Can you work these out from the model? Positions are in its coordinate system, mm. A direction names the side the tool comes from. Give positions to 0.01 mm unless a question says otherwise; leave off trailing zeros. Write each loop counter-clockwise with the first axis right and the second up, starting at its lowest first coordinate (ties: lowest second). Pieces come first, ordered by that corner, then holes. Notation, with made-up numbers: M -32,-39 L 17,-39 A24 ccw 17,-28 Z; hole C -34,79 d4. An arc over 180 degrees is marked long. Write each question's results on one line, items separated by ' | '.
from build123d import *

# Parameters (mm, degrees)
SKETCH1_W           = 101.6
SKETCH1_H           = 101.6
SKETCH1_W_2         = 4.7625
SKETCH1_H_2         = 8.89
SKETCH1_W_3         = 17.78
SKETCH1_H_3         = 50.8
SKETCH1_W_4         = 22.86
SKETCH1_H_4         = 6.35
BOSS_EXTRUDE1_DEPTH = 4.7625
FILLET1_R           = 5.08


with BuildPart() as part:
    # Sketch1 → Boss-Extrude1 (new body)
    with BuildSketch(Plane(origin=(0, 0, 0), x_dir=(1, 0, 0), z_dir=(0, 1, 0))):
        with Locations((-50.8, 50.8)):
            Rectangle(SKETCH1_W, SKETCH1_H)
        with Locations((-94.45625, 13.335)):
            Rectangle(SKETCH1_W_2, SKETCH1_H_2, mode=Mode.SUBTRACT)
        with Locations((-94.45625, 88.265)):
            Rectangle(SKETCH1_W_2, SKETCH1_H_2, mode=Mode.SUBTRACT)
        with Locations((-71.755, 50.8)):
            Rectangle(SKETCH1_W_3, SKETCH1_H_3, mode=Mode.SUBTRACT)
        with Locations((-36.195, 81.915)):
            Rectangle(SKETCH1_W_4, SKETCH1_H_4, mode=Mode.SUBTRACT)
        with Locations((-7.14375, 13.335)):
            Rectangle(SKETCH1_W_2, SKETCH1_H_2, mode=Mode.SUBTRACT)
        with Locations((-7.14375, 88.265)):
            Rectangle(SKETCH1_W_2, SKETCH1_H_2, mode=Mode.SUBTRACT)
        with Locations((-36.195, 34.925)):
            Rectangle(SKETCH1_W_4, SKETCH1_H_4, mode=Mode.SUBTRACT)
    extrude(amount=BOSS_EXTRUDE1_DEPTH)

    # Fillet1
    fillet1_edges = [part.edges().sort_by_distance(p)[0] for p in [
        (0, 2.38125, 0),
        (-101.6, 2.38125, 0),
        (-101.6, 2.38125, -101.6),
        (0, 2.38125, -101.6),
    ]]
    fillet(fillet1_edges, radius=FILLET1_R)


solid = part.part
Item 1: I want a section at A-A, the plane x = -76.5. Please give me the cut outline in (y, z), and give its area (3 significant figures).
Geometry says:
outline: M 0,-101.6 L 4.76,-101.6 L 4.76,-76.2 L 0,-76.2 Z; M 0,-25.4 L 4.76,-25.4 L 4.76,0 L 0,0 Z | area: 242 mm2
Item 2: Thinking about a two-plate mould opening in Z: for faces 3 (the face through (-72, 2, -25.4)), 4 (the face through (-1.528, 2.415, -100.151)), 5 (the face through (-51, 2, 0)), which applies, +Z half, -Z half, draft (parallel to the pull), parting line (faces both ways), or undercut?
Geometry says:
face 3: undercut | face 4: -Z half | face 5: +Z half
Item 3: I want a section at B-B, the plane x = -26. Please give me the cut outline in (y, z).
Geometry says:
outline: M 0,-101.6 L 4.76,-101.6 L 4.76,-85.09 L 0,-85.09 Z; M 0,-78.74 L 4.76,-78.74 L 4.76,-38.1 L 0,-38.1 Z; M 0,-31.75 L 4.76,-31.75 L 4.76,0 L 0,0 Z
Item 4: I want a section at D-D, the plane y = 0.95. Give the number of separate pieces and of enclosed holes in the cut face, and give its area (3 significant figures).
Geometry says:
separate pieces: 1 | enclosed holes: 7 | area: 8,940 mm2
Item 5: If I drill on line 1 (Z direction, x = -47, y = 3.45); line 2 (X direction, y = 1.9, z = -32) (3 decimals); line 3 (X direction, y = 2.65, z = -84) (1 decimal), over which ranges is the centre line in solid material (lowest first)? Write a range as from..to.
Geometry says:
line 1: z = -101.6..-85.09, -78.74..-38.1, -31.75..0 | line 2: x = -101.6..-80.645, -62.865..-47.625, -24.765..0 | line 3: x = -101.6..-96.8, -92.1..-47.6, -24.8..-9.5, -4.8..0
Item 6: I want a section at C-C, the plane z = -11.5. Please give me the cut outline in (x, y) (1 decimal), and give its area (3 significant figures).
Geometry says:
outline: M -101.6,0 L -96.8,0 L -96.8,4.8 L -101.6,4.8 Z; M -92.1,0 L -9.5,0 L -9.5,4.8 L -92.1,4.8 Z; M -4.8,0 L 0,0 L 0,4.8 L -4.8,4.8 Z | area: 439 mm2
Item 7: For faces 1 (the face through (-4.762, 2, -13)), 2 (the face through (-100.151, 2.415, -1.528)), which set-ups out of +Z, -Z, +X, -X, +Y, -Y let a thin tool reach every point of the face, with its end or its side?
Geometry says:
face 1: +Y, -Y | face 2: +Z, -X, +Y, -Y
